Print and shaded views of the part. All mm, measured from the part's lowest x, y and z. Coordinates: 2 decimals unless noted, no trailing zeros. Order: outer loops, then holes, each group sorted by start corner. A loop starts at its lowest first (then second) coordinate and runs counter-clockwise, first axis right, second up. Notation, with made-up numbers: (-19.75, -0.5) -> (30.25, -0.5) arc R34 cw to (30.25, 33.5) -> close; hole circle Ø9 at (48.5, 42.25). An arc over 180 degrees is marked (long way). Write item = value, one per line. Start each with the question number.
Q1. Cut at A-A, the plane x = 90. List the corners of the cut face in (y, z), plus the area to 3 significant figures.
Q2. Cut at C-C, the plane z = 8.5. List the corners of the cut face in (x, y), plus the area to 3 significant figures.
Q3. Cut at B-B, the plane y = 12.25. List the corners of the cut face in (x, z).
Q4. Mould opens along Y. For the marked faces 1, 2 and 3 say: +Y half, -Y half, draft (parallel to the pull), parting line (faces both ways), or undercut.
Q5. Flat gauge pins, fed straight in: pin 1 (6 mm diameter, centred on x = 90, z = 10, fed in from +Y); pin 2 (6 mm diameter, centred on x = 35, z = 10, fed in from +Y); pin 3 (12 mm diameter, centred on x = 45.5, z = 3.5, fed in from +Y). Where does each tip first touch, or does it go through?
Q6. Cut at D-D, the plane y = 2.25. List the corners of the cut face in (x, z), plus the area to 3 significant figures.
Q7. Wall check: line 1 (Z direction, x = 90, y = 2.25); line 2 (Y direction, x = 23, z = 2.5); line 3 (Y direction, x = 107, z = 8). Give the ranges that are in metal, low to high. Write a range as from..to.
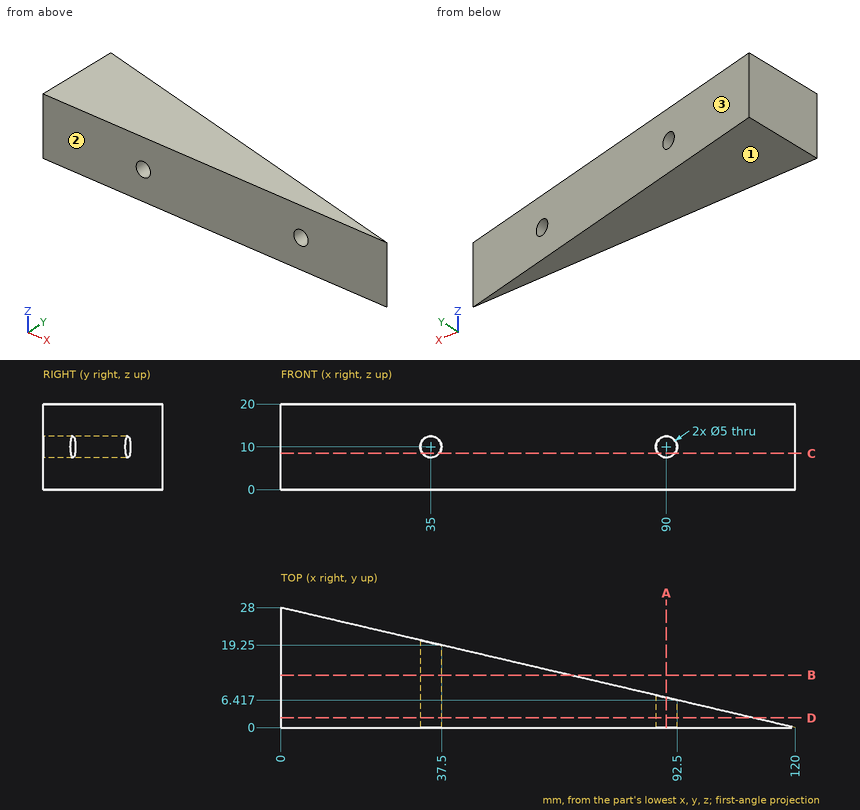
Here are the results:
q1.outline = (0, 0) -> (7, 0) -> (7, 7.5) -> (0, 7.5) -> close; (0, 12.5) -> (7, 12.5) -> (7, 20) -> (0, 20) -> close
q1.area = 105 mm²
q2.outline = (0, 0) -> (33, 0) -> (33, 20.3) -> (0, 28) -> close; (37, 0) -> (88, 0) -> (88, 7.47) -> (37, 19.37) -> close; (92, 0) -> (120, 0) -> (92, 6.53) -> close
q2.area = 1,570 mm²
q3.outline = (0, 0) -> (67.5, 0) -> (67.5, 20) -> (0, 20) -> close; hole circle Ø5 at (35, 10)
q4.face_1 = draft
q4.face_2 = -Y half
q4.face_3 = +Y half
q5.pin_1 = 7.7
q5.pin_2 = 20.53
q5.pin_3 = 18.78
q6.outline = (0, 0) -> (110.36, 0) -> (110.36, 20) -> (0, 20) -> close; hole circle Ø5 at (35, 10); hole circle Ø5 at (90, 10)
q6.area = 2,170 mm²
q7.line_1 = 0..7.5, 12.5..20
q7.line_2 = 0..22.63
q7.line_3 = 0..3.03
